Can you work these out from the model? Positions are in its coordinate system, mm. Face numbers are marked on the shaded views. Round coordinates to 2 decimals unless told otherwise and drop trailing zeros. Loops run counter-clockwise (first coordinate to the right, second up) from the corner with the lowest first, then second, coordinate; pieces in that order, holes last. Notation, with made-up numbers: (57.25, -28) - (95.25, -28) arc R23 cw to (95.25, -14) - close; hole circle Ø11 at (46.25, 39). An arc over 180 degrees is marked (long way). Answer as CSV lines item,"result".
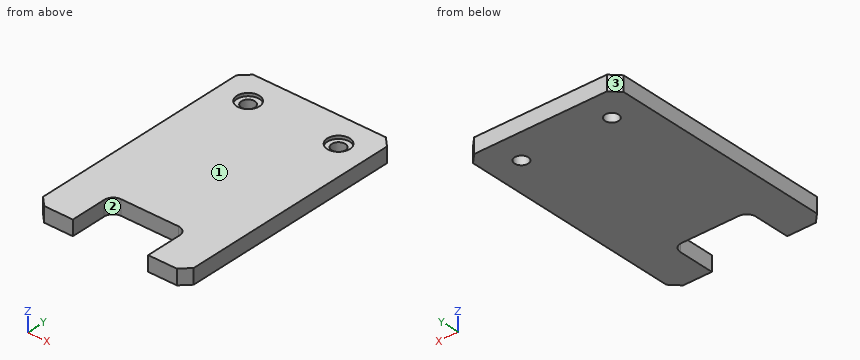
```python
from build123d import *

# Parameters (mm, degrees)
F0_W     = 50
F0_H     = 80
F1_DEPTH = 5
F2_W     = 25
F2_H     = 15
F3_DEPTH = 25
F4_R     = 3
F6_SIZE  = 3
F7_D     = 4.5
F7_DEPTH = 12
F5_R     = 3.75
F8_DEPTH = 1


with BuildPart() as f1:
    # F0 (on Top) → F1 (new body)
    with BuildSketch(Plane.XY):
        with Locations((25, 40)):
            Rectangle(F0_W, F0_H)
    extrude(amount=F1_DEPTH)

    # F2 (on face) → F3 (cut)
    with BuildSketch(Plane.XY.offset(5)):
        with Locations((25, 7.5)):
            Rectangle(F2_W, F2_H)
    extrude(amount=-F3_DEPTH, mode=Mode.SUBTRACT)

    # F4
    f4_edges = [f1.edges().sort_by_distance(p)[0] for p in [
        (12.5, 15, 2.5),
        (37.5, 15, 2.5),
    ]]
    fillet(f4_edges, radius=F4_R)

    # F6
    f6_edges = [f1.edges().sort_by_distance(p)[0] for p in [
        (0, 80, 2.5),
        (50, 80, 2.5),
        (0, 0, 2.5),
        (50, 0, 2.5),
    ]]
    chamfer(f6_edges, length=F6_SIZE)

    # F7
    with Locations(Plane.XY.offset(5)):
        with Locations((10, 70), (40, 70)):
            Hole(F7_D / 2, depth=F7_DEPTH)

    # F5 (on face) → F8 (cut)
    with BuildSketch(Plane.XY.offset(5)):
        with Locations((10, 70)):
            Circle(F5_R)
        with Locations((40, 70)):
            Circle(F5_R)
    extrude(amount=-F8_DEPTH, mode=Mode.SUBTRACT)


solid = f1.part
```
Q1. I'm going to push flat-ended pins straight in: pin 1 Ø4 at (x, y) = (9.5, 69) entering from +Z; pin 2 Ø3.5 at (x, y) = (40, 70) entering from +Z; pin 3 Ø12 at (x, y) = (40, 70) entering from +Z. Where does each tip first touch, or does it pass through?
Checks:
pin 1,"z = 4"
pin 2,"through"
pin 3,"z = 5"
Q2. If I drill on line 1 along X through (y, z) = (7, 0.55); line 2 along Y through (x, z) = (40, 2.05); line 3 along Y through (x, z) = (10, 4.4), over which ranges is the centre line in solid material (lowest first)? Write a range as [from, to].
Checks:
line 1,"[0, 12.5], [37.5, 50]"
line 2,"[0, 67.75], [72.25, 80]"
line 3,"[0, 66.25], [73.75, 80]"
Q3. Imagine slicing it at D-D (x = 20). Write out the boundary of the cut face in (y, z).
Checks:
outline,"(15, 0) - (80, 0) - (80, 5) - (15, 5) - close"
Q4. Imagine slicing it at B-B (y = 70). Write out the boundary of the cut face in (x, z).
Checks:
outline,"(0, 0) - (7.75, 0) - (7.75, 4) - (6.25, 4) - (6.25, 5) - (0, 5) - close; (12.25, 0) - (37.75, 0) - (37.75, 4) - (36.25, 4) - (36.25, 5) - (13.75, 5) - (13.75, 4) - (12.25, 4) - close; (42.25, 0) - (50, 0) - (50, 5) - (43.75, 5) - (43.75, 4) - (42.25, 4) - close"
Q5. We'd pull the mould along X, two halves only. Please class the marked faces 1, 2 and 3: pulls with the +X half, pulls with the -X half, needs draft (parallel to the pull), parting line crosses it, or undercut.
Checks:
face 1,"needs draft"
face 2,"undercut"
face 3,"pulls with the -X half"
Q6. Imagine slicing it at A-A (z = 1.8). Write out the boundary of the cut face in (x, y).
Checks:
outline,"(0, 3) - (3, 0) - (12.5, 0) - (12.5, 12) arc R3 cw to (15.5, 15) - (34.5, 15) arc R3 cw to (37.5, 12) - (37.5, 0) - (47, 0) - (50, 3) - (50, 77) - (47, 80) - (3, 80) - (0, 77) - close; hole circle Ø4.5 at (10, 70); hole circle Ø4.5 at (40, 70)"
Q7. Imagine slicing it at C-C (x = 10). Write out the boundary of the cut face in (y, z).
Checks:
outline,"(0, 0) - (67.75, 0) - (67.75, 4) - (66.25, 4) - (66.25, 5) - (0, 5) - close; (72.25, 0) - (80, 0) - (80, 5) - (73.75, 5) - (73.75, 4) - (72.25, 4) - close"
